Geometry: final body of the model. Coordinates: model frame, mm. Face numbers are marked on the shaded views. A direction names the side the tool comes from. Coordinates: 2 decimals unless noted, no trailing zeros. Order: outer loops, then holes, each group sorted by start corner. A loop starts at its lowest first (then second) coordinate and runs counter-clockwise, first axis right, second up. Notation, with made-up numbers: (-39.75, 70) -> (1.25, 70) arc R30 cw to (1.25, 100) -> close; hole circle Ø11 at (29, -36.5). An arc over 180 degrees is marked (long way). Use CSV: the item, a comma, the result in double quotes. Start each with the question number.
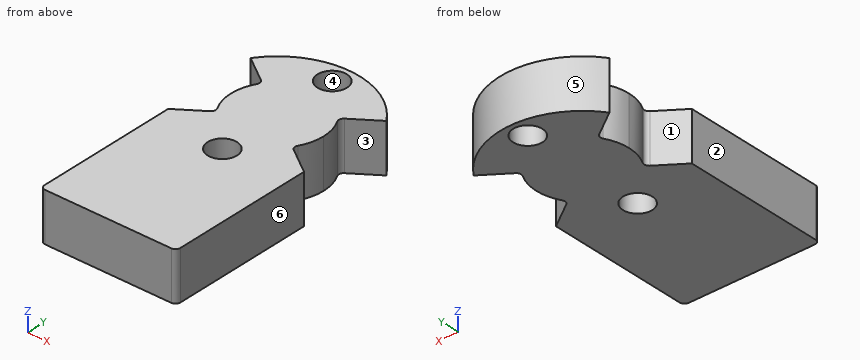
from build123d import *

# Parameters (mm, degrees)
SKETCH_1_R          = 8.5
EXTRUDE_1_DEPTH     = 5
SKETCH_2_R          = 1.5
CUT_EXTRUDE_1_DEPTH = 5
CUT_EXTRUDE_2_DEPTH = 6
EXTRUDE_2_DEPTH     = 5
FILLET_1_R          = 0.5
FILLET_2_R          = 0.5


with BuildPart() as part:
    # 草图1 → 凸台-拉伸1 (new body)
    with BuildSketch(Plane.XY):
        Circle(SKETCH_1_R)
    extrude(amount=EXTRUDE_1_DEPTH)

    # 草图2 → 切除-拉伸1 (cut)
    with BuildSketch(Plane.XY.offset(5)):
        with Locations((0, 6.5)):
            Circle(SKETCH_2_R)
        with Locations((0, -6.5)):
            Circle(SKETCH_2_R)
    extrude(amount=-CUT_EXTRUDE_1_DEPTH, mode=Mode.SUBTRACT)

    # 草图3 → 切除-拉伸2 (cut, through all)
    with BuildSketch(Plane(origin=(0, 0, 0), x_dir=(-1, 0, 0), z_dir=(0, 0, -1))):
        with BuildLine():
            Line((6.962792376, 4.875399709), (3.89097221, 2.724488073))
            ThreePointArc((3.89097221, 2.724488073), (4.530155516, 1.428352548), (4.75, 0))
            ThreePointArc((4.75, 0), (4.530155516, -1.428352548), (3.89097221, -2.724488073))
            Line((3.89097221, -2.724488073), (6.962792376, -4.875399709))
            ThreePointArc((6.962792376, -4.875399709), (8.106594081, -2.555999296), (8.5, 0))
            ThreePointArc((8.5, 0), (8.106594081, 2.555999296), (6.962792376, 4.875399709))
        make_face()
    cut_extrude_2 = extrude(amount=-CUT_EXTRUDE_2_DEPTH, mode=Mode.SUBTRACT)

    # 镜向1: 切除-拉伸2 across plane
    add(cut_extrude_2.mirror(Plane(origin=(0, 0, 0), x_dir=(0, 0, 1), z_dir=(1, 0, 0))), mode=Mode.SUBTRACT)


with BuildPart() as body_2:
    # 草图4 → 凸台-拉伸2 (new body)
    with BuildSketch(Plane(origin=(0, 0, 0), x_dir=(-1, 0, 0), z_dir=(0, 0, -1))):
        with BuildLine():
            ThreePointArc((6.962792376, -4.875399709), (0, -8.5), (-6.962792376, -4.875399709))
            Line((-6.962792376, -4.875399709), (-6.962792376, -20))
            Line((-6.962792376, -20), (6.962792376, -20))
            Line((6.962792376, -20), (6.962792376, -4.875399709))
        make_face()
    extrude(amount=-EXTRUDE_2_DEPTH)


with BuildPart() as part_1:
    add(part.part)

    # Combine 1: union body 2
    add(body_2.part)

    # 圆角1
    fillet_1_edges = [part_1.edges().sort_by_distance(p)[0] for p in [
        (-3.89097221, -2.724488073, 2.5),
        (-3.89097221, 2.724488073, 2.5),
        (3.89097221, 2.724488073, 2.5),
        (3.89097221, -2.724488073, 2.5),
    ]]
    fillet(fillet_1_edges, radius=FILLET_1_R)

    # 圆角2
    fillet_2_edges = [part_1.edges().sort_by_distance(p)[0] for p in [
        (-6.962792376, -20, 2.5),
        (6.962792376, -20, 2.5),
    ]]
    fillet(fillet_2_edges, radius=FILLET_2_R)


solid = part_1.part
(1) Section B-B (x = 0). Return loops of the section in (y, z).
(2) Section C-C (z = 0.75). Return loops of the section in (x, y), then the cut area to 3 significant figures.
(3) First-contact query: pin 1 (3 mm diameter, centred on x = 3.5, y = 1.5, fed in from -Z); pin 2 (1 mm diameter, centred on x = 4.5, z = 2, fed in from +Y). Flat tips, straight axial feed; report the tip coordinate or a pass-through.
(4) Section D-D (x = -5.25). Return loops of the section in (y, z), then the cut area to 3 significant figures.
(5) Access query for the marked faces 1, 2 and 3. Directions: +Z, -Z, +X, -X, +Y, -Y. A direction counts if a zero-diameter tool reaches every point of the face in a straight line with its end or side. Return the directions, or none.
(6) Line query: line 1 (Y direction, x = 0, z = 2.15); line 2 (Y direction, x = 5.5, z = 3.7); line 3 (Y direction, x = 3, z = 0.6). Output: solid intervals per line, ascending. Write a range as from..to.
(7) Section A-A (y = -6.5). Return loops of the section in (x, z).
(8) Mould query, pull axis Y, two halves, no side actions, for the marked faces 4, 5 and 6. Classes: pulls with the +Y half, pulls with the -Y half, needs draft (parallel to the pull), parting line crosses it, or undercut.
Check sheet entries:
1,outline,"(-20, 0) -> (-8, 0) -> (-8, 5) -> (-20, 5) -> close; (-5, 0) -> (5, 0) -> (5, 5) -> (-5, 5) -> close; (8, 0) -> (8.5, 0) -> (8.5, 5) -> (8, 5) -> close"
2,outline,"(-6.96, -19.5) arc R0.5 ccw to (-6.46, -20) -> (6.46, -20) arc R0.5 ccw to (6.96, -19.5) -> (6.96, -4.88) -> (4.28, -3) arc R0.5 cw to (4.13, -2.34) arc R4.75 ccw to (4.13, 2.34) arc R0.5 cw to (4.28, 3) -> (6.96, 4.88) arc R8.5 ccw to (-6.96, 4.88) -> (-4.28, 3) arc R0.5 cw to (-4.13, 2.34) arc R4.75 ccw to (-4.13, -2.34) arc R0.5 cw to (-4.28, -3) -> (-6.96, -4.88) -> close; hole circle Ø3 at (0, -6.5); hole circle Ø3 at (0, 6.5)"
2,area,"327 mm^2"
3,pin 1,"stops at z = 0"
3,pin 2,"stops at y = 7.5"
4,outline,"(-20, 0) -> (-3.68, 0) -> (-3.68, 5) -> (-20, 5) -> close; (3.68, 0) -> (6.68, 0) -> (6.68, 5) -> (3.68, 5) -> close"
4,area,"96.7 mm^2"
5,face 1,"+Z, -Z, -X"
5,face 2,"+Z, -Z, -X, +Y, -Y"
5,face 3,"+Z, -Z, +X"
6,line 1,"y = -20..-8, -5..5, 8..8.5"
6,line 2,"y = -20..-3.85, 3.85..6.48"
6,line 3,"y = -20..7.95"
7,outline,"(-6.96, 0) -> (-1.5, 0) -> (-1.5, 5) -> (-6.96, 5) -> close; (1.5, 0) -> (6.96, 0) -> (6.96, 5) -> (1.5, 5) -> close"
8,face 4,"undercut"
8,face 5,"pulls with the +Y half"
8,face 6,"needs draft"
